Could you check a few things on this model? Use its own coordinates, in mm. Face numbers are marked on the shaded views. A direction names the side the tool comes from. Round coordinates to 2 decimals unless told otherwise and drop trailing zeros. Loops run counter-clockwise (first coordinate to the right, second up) from the corner with the lowest first, then second, coordinate; pieces in that order, holes last. Notation, with made-up numbers: (21.25, 39.5) -> (79.25, 39.5) arc R29 cw to (79.25, 68.5) -> close; hole circle Ø2 at (27, 72.5). An arc over 180 degrees is marked (long way). Put each result on its own line as item: value. Start each with the question number.
1. I'm going to push flat-ended pins straight in: P1, Ø7, axis at y = -17.5, z = 10, coming from the +X side; P2, Ø2, axis at y = -20.5, z = 14.5, coming from the -X side; P3, Ø12, axis at x = 3.5, y = -16, coming from the +Z side. Where does each tip first touch, or does it pass through?
2. If we mould it in two halves opening along X, with no side actions, what happens to the marked faces 4, 5, 6 and 7? For each: pulls with the +X half, pulls with the -X half, needs draft (parallel to the pull), parting line crosses it, or undercut.
3. I need wall thicknesses on line 1 (X direction, y = -21.5, z = 14.5); line 2 (Y direction, x = -5, z = 3.25); line 3 (Y direction, x = -7.75, z = 14). Which ranges of each line are inside material? Lowest first, please. Write a range as [from, to].
4. Imagine slicing it at B-B, the plane x = -7. Please give me the cut outline in (y, z), and give its area (3 significant figures).
5. Imagine slicing it at D-D, the plane z = 6.25. Please give me the cut outline in (x, y), and give its area (3 significant figures).
6. Imagine slicing it at C-C, the plane z = 14. Please give me the cut outline in (x, y).
7. Imagine slicing it at A-A, the plane y = -7.5. Please give me the cut outline in (x, z), and give its area (3 significant figures).
8. Which directions (+Z, -Z, +X, -X, +Y, -Y) give clear straight access to the entire face, cutting with the end or side of a thin tool? Please do the marked faces 1, 2 and 3.
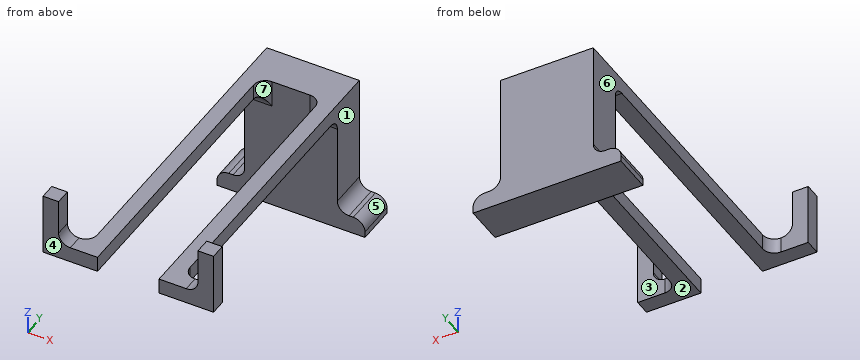
```python
from build123d import *

# Parameters (mm, degrees)
BOSS_EXTRUDE1_DEPTH = 5
SKETCH2_W           = 2
SKETCH2_H           = 2
BOSS_EXTRUDE2_DEPTH = 37
SKETCH3_W           = 2
SKETCH3_H           = 2
BOSS_EXTRUDE3_DEPTH = 5
SKETCH4_W           = 2
SKETCH4_H           = 2
BOSS_EXTRUDE4_DEPTH = 5
SKETCH5_W           = 2
SKETCH5_H           = 2
BOSS_EXTRUDE5_DEPTH = 6
FILLET2_R           = 1.5
FILLET3_R           = 1.5


with BuildPart() as part:
    # Sketch1 → Boss-Extrude1 (new body)
    with BuildSketch(Plane(origin=(0, 0, 0), x_dir=(1, 0, 0), z_dir=(0, 1, 0))):
        Polygon((-9.5, 2.3), (9.5, 2.3), (9.5, 0), (5.95, 0), (5.95, -15.3), (-5.95, -15.3), (-5.95, 0), (-9.5, 0), align=None)
    extrude(amount=BOSS_EXTRUDE1_DEPTH)

    # Sketch2 → Boss-Extrude2 (add)
    with BuildSketch(Plane.XZ):
        with Locations((-4.95, 14.3)):
            Rectangle(SKETCH2_W, SKETCH2_H)
        with Locations((4.95, 14.3)):
            Rectangle(SKETCH2_W, SKETCH2_H)
    extrude(amount=BOSS_EXTRUDE2_DEPTH)

    # Sketch3 → Boss-Extrude3 (add)
    with BuildSketch(Plane.ZY.offset(5.95)):
        with Locations((14.3, -36)):
            Rectangle(SKETCH3_W, SKETCH3_H)
    extrude(amount=BOSS_EXTRUDE3_DEPTH)

    # Sketch4 → Boss-Extrude4 (add)
    with BuildSketch(Plane(origin=(5.95, 0, 0), x_dir=(0, 0, -1), z_dir=(1, 0, 0))):
        with Locations((-14.3, -36)):
            Rectangle(SKETCH4_W, SKETCH4_H)
    extrude(amount=BOSS_EXTRUDE4_DEPTH)

    # Sketch5 → Boss-Extrude5 (add)
    with BuildSketch(Plane.XY.offset(15.3)):
        with Locations((-9.95, -36)):
            Rectangle(SKETCH5_W, SKETCH5_H)
        with Locations((9.95, -36)):
            Rectangle(SKETCH5_W, SKETCH5_H)
    extrude(amount=BOSS_EXTRUDE5_DEPTH)

    # Fillet2
    fillet2_edges = [part.edges().sort_by_distance(p)[0] for p in [
        (9.5, 2.5, 0),
        (5.95, 2.5, 0),
        (-5.95, 2.5, 0),
        (-9.5, 2.5, 0),
        (-4.95, 0, 13.3),
        (-3.95, 0, 14.3),
        (3.95, 0, 14.3),
        (4.95, 0, 13.3),
        (-5.95, -35, 14.3),
        (5.95, -35, 14.3),
    ]]
    fillet(fillet2_edges, radius=FILLET2_R)

    # Fillet3
    fillet3_edges = [part.edges().sort_by_distance(p)[0] for p in [
        (-8.95, -36, 15.3),
        (8.95, -36, 15.3),
    ]]
    fillet(fillet3_edges, radius=FILLET3_R)


solid = part.part
```
Entries:
1. P1: x = 5.95
1. P2: x = -5.95
1. P3: z = 15.3
2. face 4: needs draft
2. face 5: pulls with the +X half
2. face 6: pulls with the -X half
2. face 7: undercut
3. line 1: [-5.95, -3.95], [3.95, 5.95]
3. line 2: [0, 5]
3. line 3: [-37, -35]
4. outline: (-37, 13.3) -> (-34.93, 13.3) -> (-34.93, 15.3) -> (-37, 15.3) -> close; (0, -2.3) -> (5, -2.3) -> (5, 0.07) -> (0, 0.07) -> close
4. area: 16.0 mm^2
5. outline: (-5.95, 0) -> (5.95, 0) -> (5.95, 5) -> (-5.95, 5) -> close
5. area: 59.5 mm^2
6. outline: (-10.95, -37) -> (-3.95, -37) -> (-3.95, -1.5) arc R1.5 cw to (-2.45, 0) -> (2.45, 0) arc R1.5 cw to (3.95, -1.5) -> (3.95, -37) -> (10.95, -37) -> (10.95, -35) -> (7.45, -35) arc R1.5 cw to (5.95, -33.5) -> (5.95, 5) -> (-5.95, 5) -> (-5.95, -33.5) arc R1.5 cw to (-7.45, -35) -> (-10.95, -35) -> close
7. outline: (-5.95, 13.3) -> (-3.95, 13.3) -> (-3.95, 15.3) -> (-5.95, 15.3) -> close; (3.95, 13.3) -> (5.95, 13.3) -> (5.95, 15.3) -> (3.95, 15.3) -> close
7. area: 8.00 mm^2
8. face 1: +Z, +X, +Y
8. face 2: -Z, +X, -X, -Y
8. face 3: +Z, -Z, +X, +Y
